from build123d import *

# Parameters (mm, degrees)
SKETCH1_W           = 15
SKETCH1_H           = 15
SKETCH1_R           = 2.7
BOSS_EXTRUDE1_DEPTH = 5
BOSS_EXTRUDE2_START = 3
SKETCH1_3_W         = 15
SKETCH1_3_H         = 15
SKETCH1_3_R         = 2.7
BOSS_EXTRUDE2_DEPTH = 3
CHAMFER1_SIZE       = 5


with BuildPart() as part:
    # Sketch1 → Boss-Extrude1 (new body)
    # profile 1 of 3: a face of its own
    with BuildSketch(Plane(origin=(0, 0, 0), x_dir=(1, 0, 0), z_dir=(0, 1, 0))):
        Rectangle(SKETCH1_W, SKETCH1_H)
        Circle(SKETCH1_R, mode=Mode.SUBTRACT)
    # profile 2 of 3: a face of its own
    with BuildSketch(Plane(origin=(0, 0, 0), x_dir=(1, 0, 0), z_dir=(0, 1, 0))):
        with BuildLine():
            ThreePointArc((2.097617696, 1.7), (0, 2.7), (-2.097617696, 1.7))
            Line((-2.097617696, 1.7), (2.097617696, 1.7))
        make_face()
    # profile 3 of 3: a face of its own
    with BuildSketch(Plane(origin=(0, 0, 0), x_dir=(1, 0, 0), z_dir=(0, 1, 0))):
        with BuildLine():
            Line((2.097617696, -1.7), (-2.097617696, -1.7))
            ThreePointArc((-2.097617696, -1.7), (0, -2.7), (2.097617696, -1.7))
        make_face()
    extrude(amount=-BOSS_EXTRUDE1_DEPTH)

    # Sketch1<3> → Boss-Extrude2 (add)
    # profile 1 of 4: a face of its own
    with BuildSketch(Plane(origin=(0, 0, 0), x_dir=(1, 0, 0), z_dir=(0, 1, 0)).offset(BOSS_EXTRUDE2_START)):
        Rectangle(SKETCH1_3_W, SKETCH1_3_H)
        Circle(SKETCH1_3_R, mode=Mode.SUBTRACT)
    # profile 2 of 4: a face of its own
    with BuildSketch(Plane(origin=(0, 0, 0), x_dir=(1, 0, 0), z_dir=(0, 1, 0)).offset(BOSS_EXTRUDE2_START)):
        with BuildLine():
            ThreePointArc((2.097617696, 1.7), (0, 2.7), (-2.097617696, 1.7))
            Line((-2.097617696, 1.7), (2.097617696, 1.7))
        make_face()
    # profile 3 of 4: a face of its own
    with BuildSketch(Plane(origin=(0, 0, 0), x_dir=(1, 0, 0), z_dir=(0, 1, 0)).offset(BOSS_EXTRUDE2_START)):
        with BuildLine():
            Line((2.097617696, 1.7), (-2.097617696, 1.7))
            ThreePointArc((-2.097617696, 1.7), (-2.7, 0), (-2.097617696, -1.7))
            Line((-2.097617696, -1.7), (2.097617696, -1.7))
            ThreePointArc((2.097617696, -1.7), (2.54495263, -0.901784958), (2.7, 0))
            ThreePointArc((2.7, 0), (2.54495263, 0.901784958), (2.097617696, 1.7))
        make_face()
    # profile 4 of 4: a face of its own
    with BuildSketch(Plane(origin=(0, 0, 0), x_dir=(1, 0, 0), z_dir=(0, 1, 0)).offset(BOSS_EXTRUDE2_START)):
        with BuildLine():
            Line((2.097617696, -1.7), (-2.097617696, -1.7))
            ThreePointArc((-2.097617696, -1.7), (0, -2.7), (2.097617696, -1.7))
        make_face()
    extrude(amount=-BOSS_EXTRUDE2_DEPTH)

    # Chamfer1
    # the kernel refuses this chamfer: 5 mm, written as the material it takes off along each edge
    with BuildSketch(Plane(origin=(-7.5, -5, 20.35841494), x_dir=(-0.027495876610586317, 0.9996219169112968, 0), z_dir=(0, 0, -1)), Plane(origin=(7.5, -5, -20.35841494), x_dir=(0.027495876610586317, 0.9996219169112968, 0), z_dir=(0, 0, 1)), Plane(origin=(-20.35841494, -5, -7.5), x_dir=(0, 0.9996219169112968, -0.027495876610586317), z_dir=(1, 0, 0))) as chamfer1_piece_1:
        Polygon((CHAMFER1_SIZE * 0.999621916911, CHAMFER1_SIZE * 0.0274958766106), (-CHAMFER1_SIZE * 0.0274958766106, CHAMFER1_SIZE * 0.999621916911), (0, 0), align=None)
    extrude(amount=40.71682988, mode=Mode.SUBTRACT)
    with BuildSketch(Plane(origin=(20.35841494, -5, 7.5), x_dir=(0, -0.027495876610586317, -0.9996219169112968), z_dir=(-1, 0, 0))) as chamfer1_piece_2:
        Polygon((CHAMFER1_SIZE * 0.999621916911, -CHAMFER1_SIZE * 0.0274958766106), (-CHAMFER1_SIZE * 0.0274958766106, -CHAMFER1_SIZE * 0.999621916911), (0, 0), align=None)
    extrude(amount=40.71682988, mode=Mode.SUBTRACT)


solid = part.part
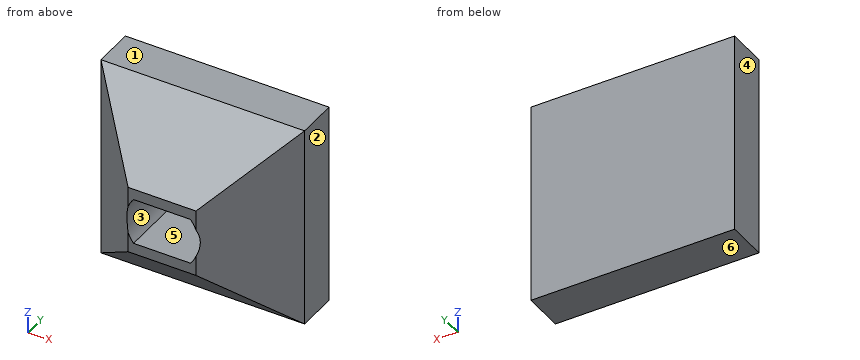
Here's how the part is built. I have some questions about the finished solid (model axes, mm). Face numbers are marked on the shaded views. A direction names the side the tool comes from. Give positions to 0.01 mm unless a question says otherwise; leave off trailing zeros. Order: outer loops, then holes, each group sorted by start corner. A loop starts at its lowest first (then second) coordinate and runs counter-clockwise, first axis right, second up. Notation, with made-up numbers: (5, 24.25) -> (21, 24.25) arc R30 cw to (21, 54.25) -> close; hole circle Ø4 at (-22.75, -13.75). An arc over 180 degrees is marked (long way). Use a Markdown table: item, result. Add a question column.
Item 1: Imagine slicing it at A-A on y = -3. Please give me the cut outline in (x, z), plus the area to 3 significant figures.
Item 2: I need wall thicknesses on line 1 (X direction, y = -3.75, z = -1.25); line 2 (Y direction, x = 1.75, z = 0.5); line 3 (Z direction, x = -1, y = -2). Which ranges of each line are inside material? Lowest first, please.
Item 3: Imagine slicing it at B-B on z = 3. Please give me the cut outline in (x, y), plus the area to 4 significant figures.
Item 4: For the marked faces 5 and 6, which set-ups out of +Z, -Z, +X, -X, +Y, -Y let a thin tool reach every point of the face, with its end or its side?
Item 5: Will these pins go through, and if not, where does the flat tip stop? pin 1 (3 mm diameter, centred on y = -2, z = -5, fed in from -X); pin 2 (2 mm diameter, centred on x = 0, y = -1.5, fed in from -Z); pin 3 (1.5 mm diameter, centred on x = -2.5, z = -5.5, fed in from -Y).
Item 6: Imagine slicing it at D-D on y = -0.5. Please give me the cut outline in (x, z), plus the area to 3 significant figures.
Item 7: Imagine slicing it at C-C on x = -5. Please give me the cut outline in (y, z).
Item 8: If we mould it in two halves opening along X, with no side actions, what happens to the marked faces 1, 2, 3 and 4? For each: pulls with the +X half, pulls with the -X half, needs draft (parallel to the pull), parting line crosses it, or undercut.
Data:
| question | item | result |
|---|---|---|
| 1 | outline | (-4.5, -4.5) -> (4.5, -4.5) -> (4.5, 4.5) -> (-4.5, 4.5) -> close; hole (-2.1, -1.7) -> (2.1, -1.7) arc R2.7 ccw to (2.1, 1.7) -> (-2.1, 1.7) arc R2.7 ccw to start |
| 1 | area | 63.9 mm² |
| 2 | line 1 | x = -3.75 to -2.39, 2.39 to 3.75 |
| 2 | line 2 | y = 0 to 3 |
| 2 | line 3 | z = -5.5 to -1.7, 1.7 to 5.5 |
| 3 | outline | (-7.5, 0) -> (-3, -4.5) -> (3, -4.5) -> (7.5, 0) -> (7.5, 3) -> (-7.5, 3) -> close |
| 3 | area | 92.25 mm² |
| 4 | face 5 | -Y |
| 4 | face 6 | -Z, +X, -X, +Y, -Y |
| 5 | pin 1 | stops at x = -7 |
| 5 | pin 2 | stops at z = -7 |
| 5 | pin 3 | stops at y = -2.75 |
| 6 | outline | (-7, -7) -> (7, -7) -> (7, 7) -> (-7, 7) -> close; hole (-2.1, -1.7) -> (2.1, -1.7) arc R2.7 ccw to (2.1, 1.7) -> (-2.1, 1.7) arc R2.7 ccw to start |
| 6 | area | 179 mm² |
| 7 | outline | (-2.5, -5) -> (0, -7.5) -> (3, -7.5) -> (3, 7.5) -> (0, 7.5) -> (-2.5, 5) -> close |
| 8 | face 1 | needs draft |
| 8 | face 2 | pulls with the +X half |
| 8 | face 3 | undercut |
| 8 | face 4 | pulls with the -X half |
